from build123d import *

# Parameters (mm, degrees)
F1_DEPTH = 101.6
F2_W     = 50.8
F2_H     = 38.1
F3_DEPTH = 19.05


with BuildPart() as f1:
    # F0 (on Right) → F1 (new body)
    with BuildSketch(Plane.YZ):
        Polygon((-16.204383, -15.124001), (-16.204383, -40.524001), (47.295617, -40.524001), (47.295617, 35.675999), (21.895617, 35.675999), (21.895617, -15.124001), align=None)
    extrude(amount=-F1_DEPTH)

    # F2 (on face) → F3 (cut)
    with BuildSketch(Plane.XZ.offset(-21.895617)):
        with Locations((-50.8, 16.625999)):
            Rectangle(F2_W, F2_H)
    extrude(amount=-F3_DEPTH, mode=Mode.SUBTRACT)


solid = f1.part
Geometry check sheet. Reference: the model listing, model coordinates, mm. A direction names the side the tool comes from. Coordinates: 2 decimals unless noted, no trailing zeros. Order: outer loops, then holes, each group sorted by start corner. A loop starts at its lowest first (then second) coordinate and runs counter-clockwise, first axis right, second up. Notation, with made-up numbers: (56.5, 34) - (61.5, 34) arc R16 ccw to (61.5, 55) - close; hole circle Ø8 at (-25.5, 27). An arc over 180 degrees is marked (long way). Answer in a Markdown table with one row per item. Add a question column.
1) Release check for a two-part mould opening along X. For faces 4 (the flat face through (-50, 47.296, -3)), 5 (the flat face through (-51, 31, -2.424)), 6 (the flat face through (0, 22.2, -10.4)) record: +X half, -X half, draft (parallel to the pull), parting line (faces both ways), or undercut.
2) Set-up check for faces 1 (the flat face through (-50, -16.204, -28)), 2 (the flat face through (-50, 21.896, -6)), 3 (the flat face through (-51, 40.946, 17)): record each of +Z, -Z, +X, -X, +Y, -Y from which the full face is reachable in a straight line by a thin tool's end or side.
3) Cross-section at A-A, the plane x = -70.5. Record the cut outline in (y, z).
4) Cross-section at C-C, the plane y = 15. Record the cut outline in (x, z).
5) Material ranges on line 1 along Y through (x, z) = (-35, -13); line 2 along X through (y, z) = (29.5, 22); line 3 along Z through (x, y) = (-31, -9), recorded low to high. Write a range as [from, to].
6) Cross-section at B-B, the plane z = 19. Record the cut outline in (x, y).
7) Cross-section at D-D, the plane x = -11.5. Record the cut outline in (y, z).
8) Gauge pin test, flat ends, axial feed: P1, Ø19, axis at x = -46, z = 17, coming from the -Y side; P2, Ø5.5, axis at x = -38.5, y = 29, coming from the +Z side; P3, Ø1, axis at x = -27.5, y = 0.5, coming from the +Z side. Record the tip position at first contact, or that the pin passes through.
Check result:
| question | item | result |
|---|---|---|
| 1 | face 4 | draft |
| 1 | face 5 | undercut |
| 1 | face 6 | +X half |
| 2 | face 1 | +Z, -Z, +X, -X, -Y |
| 2 | face 2 | +Z, +X, -X, -Y |
| 2 | face 3 | +Z, -Y |
| 3 | outline | (-16.2, -40.52) - (47.3, -40.52) - (47.3, 35.68) - (40.95, 35.68) - (40.95, -2.42) - (21.9, -2.42) - (21.9, -15.12) - (-16.2, -15.12) - close |
| 4 | outline | (-101.6, -40.52) - (0, -40.52) - (0, -15.12) - (-101.6, -15.12) - close |
| 5 | line 1 | y = [21.9, 47.3] |
| 5 | line 2 | x = [-101.6, -76.2], [-25.4, 0] |
| 5 | line 3 | z = [-40.52, -15.12] |
| 6 | outline | (-101.6, 21.9) - (-76.2, 21.9) - (-76.2, 40.95) - (-25.4, 40.95) - (-25.4, 21.9) - (0, 21.9) - (0, 47.3) - (-101.6, 47.3) - close |
| 7 | outline | (-16.2, -40.52) - (47.3, -40.52) - (47.3, 35.68) - (21.9, 35.68) - (21.9, -15.12) - (-16.2, -15.12) - close |
| 8 | P1 | stops at y = 40.95 |
| 8 | P2 | stops at z = -2.42 |
| 8 | P3 | stops at z = -15.12 |
